from build123d import *

# Parameters (mm, degrees)
DODANIE_WYCI_GNI_CIE1_DEPTH = 6
SZKIC2_R                    = 4.05
WYTNIJ_WYCI_GNI_CIE1_DEPTH  = 6
SZKIC4_R                    = 4.05
WYTNIJ_WYCI_GNI_CIE4_DEPTH  = 6
WYTNIJ_WYCI_GNI_CIE5_DEPTH  = 6
SZKIC6_R                    = 4
DODANIE_WYCI_GNI_CIE2_DEPTH = 6
SZKIC7_R                    = 1.55
WYTNIJ_WYCI_GNI_CIE6_DEPTH  = 10
DODANIE_WYCI_GNI_CIE3_DEPTH = 6
WYTNIJ_WYCI_GNI_CIE7_DEPTH  = 6


with BuildPart() as part:
    # Szkic1 → Dodanie-wyciągnięcie1 (new body)
    with BuildSketch(Plane.XY):
        with BuildLine():
            Line((183.434880274, 83.617157096), (183.434880274, 42.242261437))
            ThreePointArc((183.434880274, 42.242261437), (183.264795483, 39.639481612), (182.757433993, 37.080971114))
            Line((182.757433993, 37.080971114), (167.434880274, -20.282759431))
            Line((167.434880274, -20.282759431), (152.500436986, -16.293587051))
            Line((152.500436986, -16.293587051), (166.757433993, 37.080971114))
            ThreePointArc((166.757433993, 37.080971114), (167.264795483, 39.639481612), (167.434880274, 42.242261437))
            Line((167.434880274, 42.242261437), (167.434880274, 83.617157096))
            Line((167.434880274, 83.617157096), (183.434880274, 83.617157096))
        make_face()
    extrude(amount=DODANIE_WYCI_GNI_CIE1_DEPTH)

    # Szkic2 → Wytnij-wyciągnięcie1 (cut)
    with BuildSketch(Plane.XY.offset(6)):
        with Locations((175.434880274, 39.617157096)):
            Circle(SZKIC2_R)
        with Locations((175.434880274, -14.382842904)):
            Circle(SZKIC2_R)
    extrude(amount=-WYTNIJ_WYCI_GNI_CIE1_DEPTH, mode=Mode.SUBTRACT)

    # Szkic4 → Wytnij-wyciągnięcie4 (cut)
    with BuildSketch(Plane.XY.offset(6)):
        with Locations((161.770374916, -10.489221815)):
            Circle(SZKIC4_R)
    extrude(amount=-WYTNIJ_WYCI_GNI_CIE4_DEPTH, mode=Mode.SUBTRACT)

    # Szkic5 → Wytnij-wyciągnięcie5 (cut)
    with BuildSketch(Plane.XY.offset(6)):
        with BuildLine():
            Line((167.434880274, 73.777889147), (167.434880274, 83.617157096))
            Line((167.434880274, 83.617157096), (179.126801066, 83.617157096))
            ThreePointArc((179.126801066, 83.617157096), (171.51222692, 80.799152225), (167.434880274, 73.777889147))
        make_face()
    extrude(amount=-WYTNIJ_WYCI_GNI_CIE5_DEPTH, mode=Mode.SUBTRACT)

    # Szkic6 → Dodanie-wyciągnięcie2 (add)
    with BuildSketch(Plane.XY.offset(6)):
        with Locations((183.434880274, 79.617157096)):
            Circle(SZKIC6_R)
    extrude(amount=-DODANIE_WYCI_GNI_CIE2_DEPTH)

    # Szkic7 → Wytnij-wyciągnięcie6 (cut)
    with BuildSketch(Plane.XY.offset(6)):
        with Locations((175.434880274, 57.530770571)):
            Circle(SZKIC7_R)
        with Locations((175.434880274, 71.530770571)):
            Circle(SZKIC7_R)
    extrude(amount=-WYTNIJ_WYCI_GNI_CIE6_DEPTH, mode=Mode.SUBTRACT)

    # Szkic8 → Dodanie-wyciągnięcie3 (add)
    with BuildSketch(Plane.XY.offset(6)):
        with BuildLine():
            Line((184.768213607, 75.84592093), (183.01913403, 76.038564372))
            Line((183.01913403, 76.038564372), (183.434880274, 73.960302847))
            ThreePointArc((183.434880274, 73.960302847), (183.801887112, 75.115003385), (184.768213607, 75.84592093))
        make_face()
    extrude(amount=-DODANIE_WYCI_GNI_CIE3_DEPTH)

    # Szkic10 → Wytnij-wyciągnięcie7 (cut)
    with BuildSketch(Plane.XY.offset(6)):
        with BuildLine():
            Line((169.370364145, -13.036801787), (167.434880274, -20.282759431))
            Line((167.434880274, -20.282759431), (160.18892263, -18.34727556))
            ThreePointArc((160.18892263, -18.34727556), (165.879478517, -17.593577473), (169.370364145, -13.036801787))
        make_face()
        with BuildLine():
            Line((154.435920857, -9.047629406), (152.500436986, -16.293587051))
            Line((152.500436986, -16.293587051), (159.74639463, -18.229070922))
            ThreePointArc((159.74639463, -18.229070922), (155.189618945, -14.738185294), (154.435920857, -9.047629406))
        make_face()
    extrude(amount=-WYTNIJ_WYCI_GNI_CIE7_DEPTH, mode=Mode.SUBTRACT)


solid = part.part
Input: part model. Units: mm. Frame: model coordinates. A direction names the side the tool comes from. Give positions to 0.01 mm unless a question says otherwise; leave off trailing zeros. Order: outer loops, then holes, each group sorted by start corner. A loop starts at its lowest first (then second) coordinate and runs counter-clockwise, first axis right, second up. Notation, with made-up numbers: M 77.25,49 L 110.25,49 A18 cw 110.25,64 Z; hole C 45,-15 d6. An arc over 180 degrees is marked long. Answer as a JSON object with one key per item and string values.
1. Cut plane C-C, the plane y = 68. Output: boundary loops of the cut face in (x, z).
Result sheet:
{"outline": "M 167.43,0 L 183.43,0 L 183.43,6 L 167.43,6 Z"}
2. Cut plane A-A, the plane x = 175. Output: boundary loops of the cut face in (y, z).
Result sheet:
{"outline": "M 8.04,0 L 35.59,0 L 35.59,6 L 8.04,6 Z; M 43.64,0 L 56.04,0 L 56.04,6 L 43.64,6 Z; M 59.02,0 L 70.04,0 L 70.04,6 L 59.02,6 Z; M 73.02,0 L 82.84,0 L 82.84,6 L 73.02,6 Z"}
3. Ray query, line 1 (X direction, y = 40.5, z = 1.35); line 2 (X direction, y = 39, z = 0.5); line 3 (X direction, y = 61, z = 5.1). Return the intervals inside material, ascending. Write a range as [from, to].
Result sheet:
{"line 1": "[167.36, 171.48], [179.39, 183.36]", "line 2": "[167.17, 171.43], [179.44, 183.17]", "line 3": "[167.43, 183.43]"}
4. Pull-direction query (Y, two-part tool) for faces 4 (the cylindrical face through (173.886, 57.599, 3.042)), 5 (the flat face through (176.158, 12.373, 2.958)), 6 (the flat face through (160.51, 13.69, 2.96)); classes: +Y half, -Y half, draft (parallel to the pull), parting line (faces both ways), or undercut.
Result sheet:
{"face 4": "undercut", "face 5": "-Y half", "face 6": "+Y half"}
5. Reachability of faces 1 (the flat face through (183.435, 58, 3)), 2 (the cylindrical face through (165.808, -17.634, 3.042)), 3 (the flat face through (167.435, 58, 3)) from +Z, -Z, +X, -X, +Y, -Y: full face, straight path, thin tool, end or side. Return the list, or none.
Result sheet:
{"face 1": "+Z, -Z, +X, -Y", "face 2": "+Z, -Z, -Y", "face 3": "+Z, -Z, -X, +Y"}
6. First-contact query: P1, Ø1.8, axis at y = 66, z = 3, coming from the +X side; P2, Ø3, axis at y = 64, z = 4, coming from the -X side; P3, Ø1.9, axis at x = 175.43, y = 57.53, coming from the +Z side. Flat tips, straight axial feed; report the tip coordinate or a pass-through.
Result sheet:
{"P1": "x = 183.43", "P2": "x = 167.43", "P3": "through"}
7. Cut plane B-B, the plane z = 1.65. Output: boundary loops of the cut face in (x, y), and give its area (3 significant figures).
Result sheet:
{"outline": "M 154.44,-9.05 A7.5 ccw 159.75,-18.23 L 160.19,-18.35 A7.5 ccw 169.37,-13.04 L 182.76,37.08 A20 ccw 183.43,42.24 L 183.43,73.96 A2 cw 184.77,75.85 A4 ccw 183.43,83.62 L 179.13,83.62 A12 ccw 167.43,73.78 L 167.43,42.24 A20 cw 166.76,37.08 Z; hole C 161.77,-10.49 d8.1; hole C 175.43,39.62 d8.1; hole C 175.43,57.53 d3.1; hole C 175.43,71.53 d3.1", "area": "1,480 mm²"}
